CAD build for the part. Positions are in the model's coordinates, mm. A direction names the side the tool comes from. Give positions to 0.01 mm unless a question says otherwise; leave off trailing zeros. Order: outer loops, then holes, each group sorted by start corner. A loop starts at its lowest first (then second) coordinate and runs counter-clockwise, first axis right, second up. Notation, with made-up numbers: M 55.25,73 L 87.25,73 A9 cw 87.25,77 Z; hole C -35,60 d8. An arc over 180 degrees is marked long. Put each result on its own line as item: value. Start each with the question number.
1) Cut at D-D (y = -13.5). Write the cut outline in (x, z), and give its area (3 significant figures).
2) Cut at A-A (z = -3.5). Write the cut outline in (x, y) (3 decimals), and give its area (3 significant figures).
3) Pin check, flat tips, straight feed: pin 1 (1.5 mm diameter, centred on y = 4.5, z = -42.5, fed in from +X); pin 2 (8 mm diameter, centred on x = 16.5, z = -9, fed in from -Y); pin 3 (7.5 mm diameter, centred on x = -27.5, z = -18.5, fed in from -Y). Stop position of each tip, or through.
4) Tool access for faces 5 (the face through (0, 0, 0)), 6 (the face through (37.162, 0.66, -99.993)), 7 (the face through (28, -21, -3)): list every direction of +Z, -Z, +X, -X, +Y, -Y with a clear straight run to the whole face (end or side of a thin tool).
5) Cut at B-B (y = 36.5). Write the cut outline in (x, z), and give its area (3 significant figures).
6) Two-plate mould, pull along Y, no slides. Class faces 1 (the face through (-29, -30, -35)), 2 (the face through (-29, 30, -35)), 3 (the face through (0, 0, -7)), 4 (the face through (44.2, -18.3, 10)): released by +Y, released by -Y, zero draft, split by the parting line, or undercut.
7) Drill centre lines: line 1 (Y direction, x = 0, z = 2.5); line 2 (X direction, y = 25, z = -5); line 3 (Z direction, x = -13.5, y = 29.5). Where is each one in solid material? Low to high. Write a range as [from, to].
8) Cut at C-C (x = -43). Write the cut outline in (y, z), and give its area (3 significant figures).
```python
from build123d import *

# Parameters (mm, degrees)
ESQUISSE1_R             = 50
BOSS_EXTRU_1_DEPTH      = 10
ESQUISSE2_R             = 47.5
ENL_V_MAT_EXTRU_1_DEPTH = 5
ESQUISSE3_R             = 2.5
ENL_V_MAT_EXTRU_2_DEPTH = 16
ESQUISSE4_R             = 35
BOSS_EXTRU_2_DEPTH      = 7
BOSS_EXTRU_3_DEPTH      = 100
CONG_1_R                = 30


with BuildPart() as part:
    # Esquisse1 → Boss.-Extru.1 (new body)
    with BuildSketch(Plane.XY):
        Circle(ESQUISSE1_R)
    extrude(amount=BOSS_EXTRU_1_DEPTH)

    # Esquisse2 → Enlèv. mat.-Extru.1 (cut)
    with BuildSketch(Plane.XY.offset(10)):
        Circle(ESQUISSE2_R)
    extrude(amount=-ENL_V_MAT_EXTRU_1_DEPTH, mode=Mode.SUBTRACT)

    # Esquisse3 → Enlèv. mat.-Extru.2 (cut)
    with BuildSketch(Plane(origin=(0, 0, 0), x_dir=(-1, 0, 0), z_dir=(0, 0, -1))):
        Circle(ESQUISSE3_R)
    extrude(amount=-ENL_V_MAT_EXTRU_2_DEPTH, mode=Mode.SUBTRACT)

    # Esquisse4 → Boss.-Extru.2 (add)
    with BuildSketch(Plane(origin=(0, 0, 0), x_dir=(-1, 0, 0), z_dir=(0, 0, -1))):
        Circle(ESQUISSE4_R)
    extrude(amount=BOSS_EXTRU_2_DEPTH)

    # Esquisse5 → Boss.-Extru.3 (add)
    with BuildSketch(Plane(origin=(0, 0, 0), x_dir=(-1, 0, 0), z_dir=(0, 0, -1))):
        with BuildLine():
            Line((-46.875, 0), (-36.875, 0))
            ThreePointArc((-36.875, 0), (-32.790583699, 16.868409696), (-21.442145998, 30))
            Line((-21.442145998, 30), (-36.017573836, 30))
            ThreePointArc((-36.017573836, 30), (-44.077144863, 15.952144863), (-46.875, 0))
        make_face()
        with BuildLine():
            ThreePointArc((-21.442145998, -30), (-32.790583699, -16.868409696), (-36.875, 0))
            Line((-36.875, 0), (-46.875, 0))
            ThreePointArc((-46.875, 0), (-44.077144863, -15.952144863), (-36.017573836, -30))
            Line((-36.017573836, -30), (-21.442145998, -30))
        make_face()
        with BuildLine():
            ThreePointArc((21.442145998, 30), (32.790583699, 16.868409696), (36.875, 0))
            Line((36.875, 0), (46.875, 0))
            ThreePointArc((46.875, 0), (44.077144863, 15.952144863), (36.017573836, 30))
            Line((36.017573836, 30), (21.442145998, 30))
        make_face()
        with BuildLine():
            Line((46.875, 0), (36.875, 0))
            ThreePointArc((36.875, 0), (32.790583699, -16.868409696), (21.442145998, -30))
            Line((21.442145998, -30), (36.017573836, -30))
            ThreePointArc((36.017573836, -30), (44.077144863, -15.952144863), (46.875, 0))
        make_face()
    extrude(amount=BOSS_EXTRU_3_DEPTH)

    # Congé1
    # the kernel refuses this fillet: 30 mm, written as the material it takes off along each edge
    with BuildSketch(Plane(origin=(-53.557854002, 30, -100), x_dir=(0, 0, 1), z_dir=(1, 0, 0)), Plane(origin=(-111.017573836, 30, -100), x_dir=(0, 0, 1), z_dir=(1, 0, 0)), Plane(origin=(111.017573836, -30, -100), x_dir=(0, 0, 1), z_dir=(-1, 0, 0)), Plane(origin=(53.557854002, -30, -100), x_dir=(0, 0, 1), z_dir=(-1, 0, 0))) as cong_1_piece_1:
        with BuildLine():
            CenterArc((CONG_1_R, CONG_1_R), CONG_1_R, 180, 90)
            Line((0, CONG_1_R), (0, 0))
            Line((0, 0), (CONG_1_R, 0))
        make_face()
    extrude(amount=164.575427838, mode=Mode.SUBTRACT)


solid = part.part
```
Solution:
1. outline: M -48.14,0 L -44.89,0 L -44.89,-96.79 L -34.31,-96.79 L -34.31,0 L -32.29,0 L -32.29,-7 L 32.29,-7 L 32.29,0 L 34.31,0 L 34.31,-96.79 L 44.89,-96.79 L 44.89,0 L 48.14,0 L 48.14,10 L 45.54,10 L 45.54,5 L -45.54,5 L -45.54,10 L -48.14,10 Z
1. area: 3,010 mm²
2. outline: M -36.018,-30 L -21.442,-30 A36.875 cw -21.442,30 L -36.018,30 A46.875 ccw Z; C 0,0 d70; M 21.442,-30 L 36.018,-30 A46.875 ccw 36.018,30 L 21.442,30 A36.875 cw Z
2. area: 5,190 mm²
3. pin 1: x = 46.72
3. pin 2: y = -32.48
3. pin 3: y = -30
4. face 5: +Z
4. face 6: -Z, +X, -X
4. face 7: -Z
5. outline: M -34.17,0 L 34.17,0 L 34.17,10 L 30.4,10 L 30.4,5 L -30.4,5 L -30.4,10 L -34.17,10 Z
5. area: 379 mm²
6. face 1: released by -Y
6. face 2: released by +Y
6. face 3: undercut
6. face 4: zero draft
7. line 1: [-50, -2.5], [2.5, 50]
7. line 2: [-39.65, -27.11], [-24.49, 24.49], [27.11, 39.65]
7. line 3: [-7, 5]
8. outline: M -25.51,0 L -18.66,0 L -18.66,-93.49 A30 ccw 18.66,-93.49 L 18.66,0 L 25.51,0 L 25.51,10 L 20.18,10 L 20.18,5 L -20.18,5 L -20.18,10 L -25.51,10 Z
8. area: 3,960 mm²
